Geometry check sheet. Reference: drawing and pictorial views, mm from the part's lowest x, y, z. Give positions to 0.01 mm unless a question says otherwise; leave off trailing zeros. Loops run counter-clockwise (first coordinate to the right, second up) from the corner with the lowest first, then second, coordinate; pieces in that order, holes last. Notation, with made-up numbers: M 52.25,-37 L 109.25,-37 A9 ccw 109.25,-31 Z; hole C 81.5,26 d7. An arc over 180 degrees is marked long. Use CSV: the item, a comma, the result in double quotes.
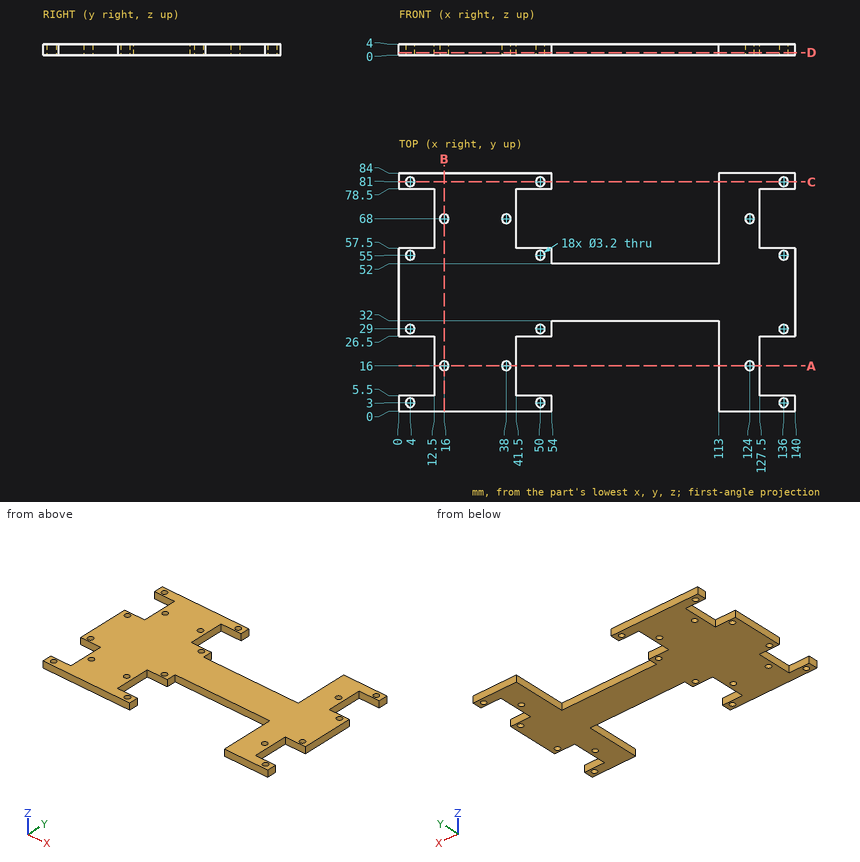
(1) Section check C-C on y = 81. Record the cut outline in (x, z).
Calculated:
outline,"M 0,0 L 2.4,0 L 2.4,4 L 0,4 Z; M 5.6,0 L 48.4,0 L 48.4,4 L 5.6,4 Z; M 51.6,0 L 54,0 L 54,4 L 51.6,4 Z; M 113,0 L 134.4,0 L 134.4,4 L 113,4 Z; M 137.6,0 L 140,0 L 140,4 L 137.6,4 Z"
(2) Section check B-B on x = 16. Record the cut outline in (y, z).
Calculated:
outline,"M 0,0 L 14.4,0 L 14.4,4 L 0,4 Z; M 17.6,0 L 66.4,0 L 66.4,4 L 17.6,4 Z; M 69.6,0 L 84,0 L 84,4 L 69.6,4 Z"
(3) Section check D-D on z = 0.95. Count the separate pieces of the cut face and the enclosed holes in it, plus the area to 3 significant figures.
Calculated:
separate pieces,"1"
enclosed holes,"18"
area,"6,260 mm²"
(4) Section check A-A on y = 16. Record the cut outline in (x, z), plus the area to 3 significant figures.
Calculated:
outline,"M 12.5,0 L 14.4,0 L 14.4,4 L 12.5,4 Z; M 17.6,0 L 36.4,0 L 36.4,4 L 17.6,4 Z; M 39.6,0 L 41.5,0 L 41.5,4 L 39.6,4 Z; M 113,0 L 122.4,0 L 122.4,4 L 113,4 Z; M 125.6,0 L 127.5,0 L 127.5,4 L 125.6,4 Z"
area,"136 mm²"
(5) Scan lines: L1, parallel to Y at x = 16, z = 2.3; L2, parallel to X at y = 68, z = 0.95; L3, parallel to Y at x = 42, z = 0.65. Record each from-to range of solid material in increasing order. Write a range as from..to.
Calculated:
L1,"y = 0..14.4, 17.6..66.4, 69.6..84"
L2,"x = 12.5..14.4, 17.6..36.4, 39.6..41.5, 113..122.4, 125.6..127.5"
L3,"y = 0..5.5, 26.5..57.5, 78.5..84"
(6) Depth check by flat-ended pin: pin 1 Ø2.5 at (x, y) = (16, 68) entering from +Z; pin 2 Ø1.2 at (y, z) = (20, 1.5) entering from +X; pin 3 Ø2 at (y, z) = (14, 1) entering from -X. Enter the tip coordinate at first touch or a pass-through.
Calculated:
pin 1,"passes through"
pin 2,"stops at x = 127.5"
pin 3,"stops at x = 12.5"
